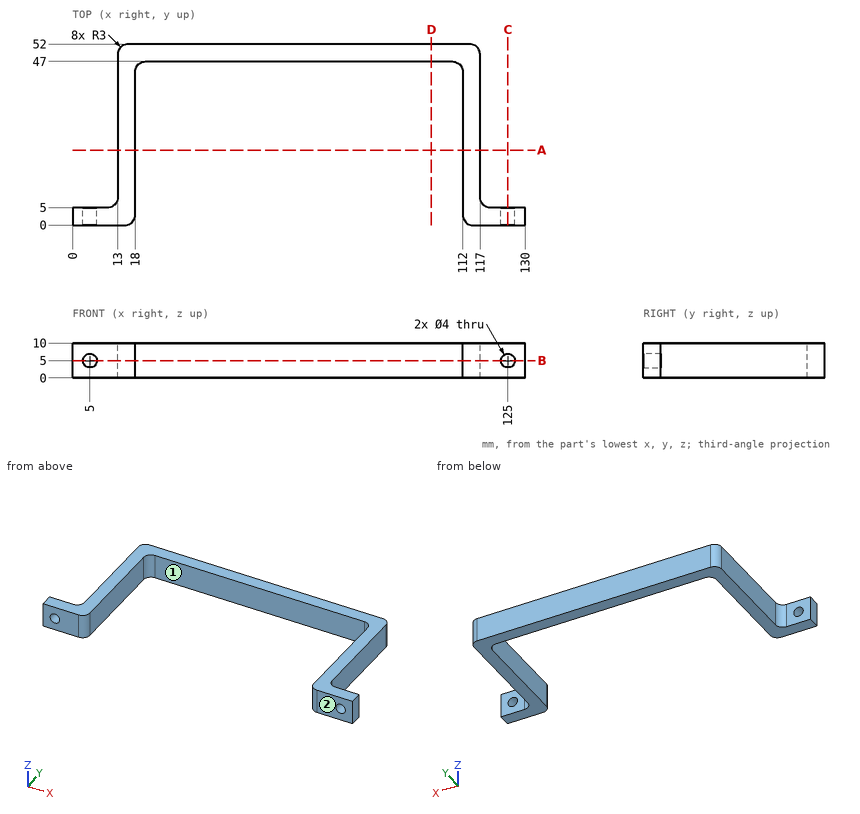
Design review of the part shown in the three views and the two pictorial views. Dimensions are in mm from the part's minimum x, y and z. Give positions to 0.01 mm unless a question says otherwise; leave off trailing zeros. Loops run counter-clockwise (first coordinate to the right, second up) from the corner with the lowest first, then second, coordinate; pieces in that order, holes last. Notation, with made-up numbers: M -1.5,-12 L 7.5,-12 A27 ccw 7.5,17 Z; hole C 0,23 d5. An arc over 180 degrees is marked long. Answer as a JSON object with one key per item and string values.
Item 1: We need section A-A (y = 21.5). State the section outline as (x, z) points.
Output values:
{"outline": "M 13,0 L 18,0 L 18,10 L 13,10 Z; M 112,0 L 117,0 L 117,10 L 112,10 Z"}
Item 2: For P1, Ø6, axis at y = 34.5, z = 3, coming from the -X side; P2, Ø3, axis at x = 59, z = 6.5, coming from the -Y side; P3, Ø2, axis at y = 38.5, z = 8.5, coming from the +X side; P4, Ø5, axis at x = 5, z = 5, coming from the -Y side, all flat-tipped, find the tip position at first contact; note any pin that passes through.
Output values:
{"P1": "stops at x = 13", "P2": "stops at y = 47", "P3": "stops at x = 117", "P4": "stops at y = 0"}
Item 3: We need section C-C (x = 125). State the section outline as (y, z) points.
Output values:
{"outline": "M 0,0 L 5,0 L 5,3 L 0,3 Z; M 0,7 L 5,7 L 5,10 L 0,10 Z"}
Item 4: We need section B-B (z = 5). State the section outline as (x, y) points, and give its area (3 significant figures).
Output values:
{"outline": "M 0,0 L 3,0 L 3,5 L 0,5 Z; M 7,0 L 15,0 A3 ccw 18,3 L 18,44 A3 cw 21,47 L 109,47 A3 cw 112,44 L 112,3 A3 ccw 115,0 L 123,0 L 123,5 L 120,5 A3 cw 117,8 L 117,49 A3 ccw 114,52 L 16,52 A3 ccw 13,49 L 13,8 A3 cw 10,5 L 7,5 Z; M 127,0 L 130,0 L 130,5 L 127,5 Z", "area": "1,080 mm2"}
Item 5: We need section D-D (x = 103). State the section outline as (y, z) points.
Output values:
{"outline": "M 47,0 L 52,0 L 52,10 L 47,10 Z"}
Item 6: Wall thickness on line 1 along X through (y, z) = (2.85, 5); line 2 along X through (y, z) = (13, 7); line 3 along X through (y, z) = (1.45, 5): over which ranges is each line inside the solid? List them lowest first.
Output values:
{"line 1": "x = 0 to 3, 7 to 18, 112 to 123, 127 to 130", "line 2": "x = 13 to 18, 112 to 117", "line 3": "x = 0 to 3, 7 to 17.57, 112.43 to 123, 127 to 130"}
Item 7: Mouldability with a two-part tool opening along X and no side actions: class the marked faces 1 and 2 as pulls with the +X half, pulls with the -X half, needs draft (parallel to the pull), parting line crosses it, or undercut.
Output values:
{"face 1": "undercut", "face 2": "needs draft"}
